Build history of the part. All positions in model axes, mm. Round coordinates to 2 decimals unless told otherwise and drop trailing zeros. Write each loop counter-clockwise with the first axis right and the second up, starting at its lowest first coordinate (ties: lowest second). Pieces come first, ordered by that corner, then holes. Notation, with made-up numbers: (52.5, 59.25) - (73.5, 59.25) arc R19 cw to (73.5, 83.25) - close; hole circle Ø1 at (84, 89.25). An arc over 180 degrees is marked (long way). One line per question, with ' | ' between items.
Autodesk Fusion 360 part; units mm, degrees
sketch "Esquisse1" plane through (0, 0, 0) normal (0, 0, 1) x (1, 0, 0)
  circle A0 centre (0, 0) radius 27.9
  circle A1 centre (0, 0) radius 28.9
  dimension "d1" = 55.8
  dimension "d2" = 57.8
extrude "Extrusion1" add sketch "Esquisse1" along normal blind 1

Autodesk Fusion 360 part; units mm, degrees
sketch "Esquisse1" plane through (0, 0, 0) normal (0, 0, 1) x (1, 0, 0)
  line L0 (-17.5, 35) -> (17.5, 35)
  line L1 (17.5, 35) -> (17.5, -35)
  line L2 (17.5, -35) -> (-17.5, -35)
  line L3 (-17.5, -35) -> (-17.5, 35)
  line L4 (-17.5, 35) -> (17.5, -35) construction
  line L5 (17.5, 35) -> (-17.5, -35) construction
  arc A0 (17.5, -35) -> (17.5, 35) centre (17.5, 0) ccw
  line L6 (-17.5, 35) -> (-12.5, 35)
  line L7 (-12.5, 35) -> (-12.5, 28)
  line L8 (-12.5, 28) -> (-17.5, 28)
  line L9 (-17.5, 28) -> (-17.5, 35)
  line L10 (-17.5, -35) -> (-12.5, -35)
  line L11 (-12.5, -35) -> (-12.5, -28)
  line L12 (-12.5, -28) -> (-17.5, -28)
  line L13 (-17.5, -28) -> (-17.5, -35)
  dimension "d1" = 35
  dimension "d2" = 70
  dimension "d13" = 7
  dimension "d14" = 5
  dimension "d15" = 5
  dimension "d16" = 7
extrude "Extrusion1" add sketch "Esquisse1" along normal blind 5 contours L0 L1 L2 L3 L7 L8 L11 L12 | L1 A0
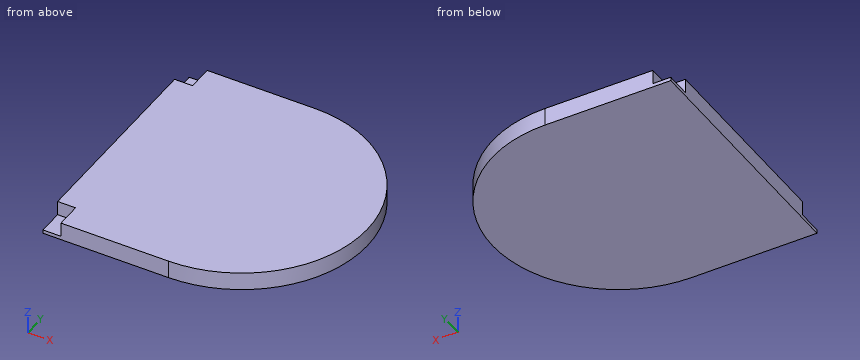
Q1. Drop flat-ended pins along their axis: pin 1 (2.5 mm diameter, centred on x = -14.5, y = -30, fed in from +Z); pin 2 (3 mm diameter, centred on x = 41.5, z = 1.5, fed in from +Y); pin 3 (2 mm diameter, centred on y = 32, z = 2.5, fed in from -X); pin 4 (6 mm diameter, centred on x = 28, y = 11, fed in from -Z). Give the stop position or say it passes through.
Found:
pin 1: z = 1 | pin 2: y = 26.81 | pin 3: x = -12.5 | pin 4: z = 0
Q2. Saw through at A-A, the plane z = 3.1. List the corners of the cut face in (x, y), then the cut area to 3 significant figures.
Found:
outline: (-17.5, -28) - (-12.5, -28) - (-12.5, -35) - (17.5, -35) arc R35 ccw to (17.5, 35) - (-12.5, 35) - (-12.5, 28) - (-17.5, 28) - close | area: 4,300 mm^2
Q3. Drill centre lines: L1, parallel to X at y = 27, z = 0.35; L2, parallel to X at y = 14, z = 4.7; L3, parallel to Y at x = 44.5, z = 4.4. Where is each one in solid material? Low to high. Write a range as from..to.
Found:
L1: -17.5..39.77 | L2: -17.5..49.58 | L3: -22.27..22.27
Q4. Saw through at C-C, the plane x = 32. List the corners of the cut face in (y, z), then the cut area to 3 significant figures.
Found:
outline: (-31.86, 0) - (31.86, 0) - (31.86, 5) - (-31.86, 5) - close | area: 319 mm^2
Q5. Saw through at D-D, the plane x = 46. List the corners of the cut face in (y, z), then the cut area to 3 significant figures.
Found:
outline: (-20.32, 0) - (20.32, 0) - (20.32, 5) - (-20.32, 5) - close | area: 203 mm^2
Q6. Saw through at B-B, the plane y = 29.5. List the corners of the cut face in (x, z).
Found:
outline: (-17.5, 0) - (36.33, 0) - (36.33, 5) - (-12.5, 5) - (-12.5, 1) - (-17.5, 1) - close
